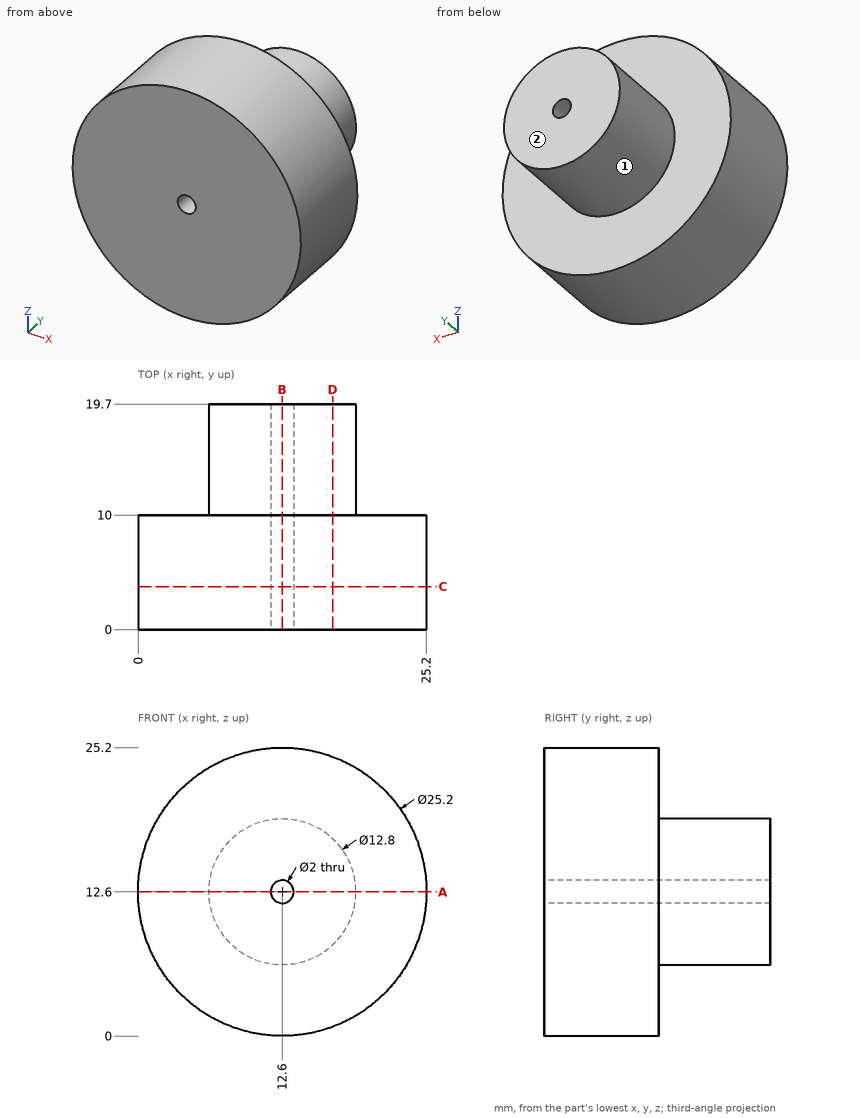
Could you check a few things on this drawing? It's one solid part, dimensions in mm from its lowest x, y, z. A direction names the side the tool comes from. Give positions to 0.01 mm unless a question says otherwise; leave off trailing zeros. Write each loop counter-clockwise with the first axis right and the second up, starting at its lowest first coordinate (ties: lowest second). Pieces come first, ordered by that corner, then holes. Notation, with made-up numbers: (44, -2) - (51, -2) arc R27 ccw to (51, 28) - close; hole circle Ø1 at (48.25, 59). An arc over 180 degrees is marked (long way). Use CSV: the item, a comma, the result in double quotes. Start each with the question number.
Item 1: I want a section at D-D, the plane x = 17. Please give me the cut outline in (y, z), then the cut area to 3 significant figures.
Item 2: I'm going to push flat-ended pins straight in: pin 1 (8 mm diameter, centred on x = 20.5, z = 5, fed in from +Y); pin 2 (1 mm diameter, centred on x = 7, y = 15, fed in from +Z); pin 3 (5 mm diameter, centred on y = 14, z = 3, fed in from -X); pin 4 (10 mm diameter, centred on x = 21.5, y = 5.5, fed in from +Z). Where does each tip first touch, or does it pass through?
Item 3: I want a section at C-C, the plane y = 3.75. Please give me the cut outline in (x, z), then the cut area to 3 significant figures.
Item 4: For the marked faces 1 and 2, which set-ups out of +Z, -Z, +X, -X, +Y, -Y let a thin tool reach every point of the face, with its end or its side?
Item 5: I want a section at B-B, the plane x = 12.6. Please give me the cut outline in (y, z), then the cut area to 3 significant figures.
Item 6: If I drill on line 1 along X through (y, z) = (7.5, 12.6); line 2 along X through (y, z) = (12.5, 12.6); line 3 along Y through (x, z) = (23, 14), over which ranges is the centre line in solid material (lowest first)?
Item 7: I want a section at A-A, the plane z = 12.6. Please give me the cut outline in (x, y), then the cut area to 3 significant figures.
Findings:
1,outline,"(0, 0.79) - (10, 0.79) - (10, 7.95) - (19.7, 7.95) - (19.7, 17.25) - (10, 17.25) - (10, 24.41) - (0, 24.41) - close"
1,area,"326 mm2"
2,pin 1,"stops at y = 10"
2,pin 2,"stops at z = 16.47"
2,pin 3,"passes through"
2,pin 4,"stops at z = 24.58"
3,outline,"circle Ø25.2 at (12.6, 12.6); hole circle Ø2 at (12.6, 12.6)"
3,area,"496 mm2"
4,face 1,"+Y"
4,face 2,"+Z, -Z, +X, -X, +Y"
5,outline,"(0, 0) - (10, 0) - (10, 6.2) - (19.7, 6.2) - (19.7, 11.6) - (0, 11.6) - close; (0, 13.6) - (19.7, 13.6) - (19.7, 19) - (10, 19) - (10, 25.2) - (0, 25.2) - close"
5,area,"337 mm2"
6,line 1,"x = 0 to 11.6, 13.6 to 25.2"
6,line 2,"x = 6.2 to 11.6, 13.6 to 19"
6,line 3,"y = 0 to 10"
7,outline,"(0, 0) - (11.6, 0) - (11.6, 19.7) - (6.2, 19.7) - (6.2, 10) - (0, 10) - close; (13.6, 0) - (25.2, 0) - (25.2, 10) - (19, 10) - (19, 19.7) - (13.6, 19.7) - close"
7,area,"337 mm2"
